The drawing under review shows one solid part. Ordinate dimensions are in mm from its lowest x, y, z. A direction names the side the tool comes from. Coordinates: 2 decimals unless noted, no trailing zeros. Write each loop counter-clockwise with the first axis right and the second up, starting at its lowest first coordinate (ties: lowest second). Pieces come first, ordered by that corner, then holes.
Q1. To check wall thickness, follow probe 1 along Y at (x, z) = (12, 112); probe 2 along Z at (x, y) = (59.3, 42). State the ranges of each line that lie inside material, in increasing order.
Q2. Add section B-B, the plane y = 42. Give the boundary of the cut face in (x, z), plus the area to 3 significant figures.
Q3. Add section A-A, the plane x = 24.5. Give the boundary of the cut face in (y, z), plus the area to 4 significant figures.
Q4. The part is to be moulded in two halves that separate along Y. For the marked faces 3, 4 and 5, say which applies: +Y half, -Y half, draft (parallel to the pull), parting line (faces both ways), or undercut.
Q5. Clearance check with flat-ended pins moving along their axes: pin 1 Ø0.9 at (x, y) = (58.5, 36) entering from -Z; pin 2 Ø2.5 at (x, y) = (28, 1.5) entering from +Z; pin 3 Ø3.5 at (x, y) = (36.5, 58.5) entering from +Z. State where each tip first meets the part, or that it passes through.
Q6. Add section D-D, the plane y = 26. Give the boundary of the cut face in (x, z).
Q7. Machinability: for the marked faces 1 and 2, which of the approach directions +Z, -Z, +X, -X, +Y, -Y give a long, thin tool a straight path to every point of the face, cutting with its end or side? Answer none if there is none.
Q8. Add section C-C, the plane z = 35. Give the boundary of the cut face in (x, y), plus the area to 3 significant figures.
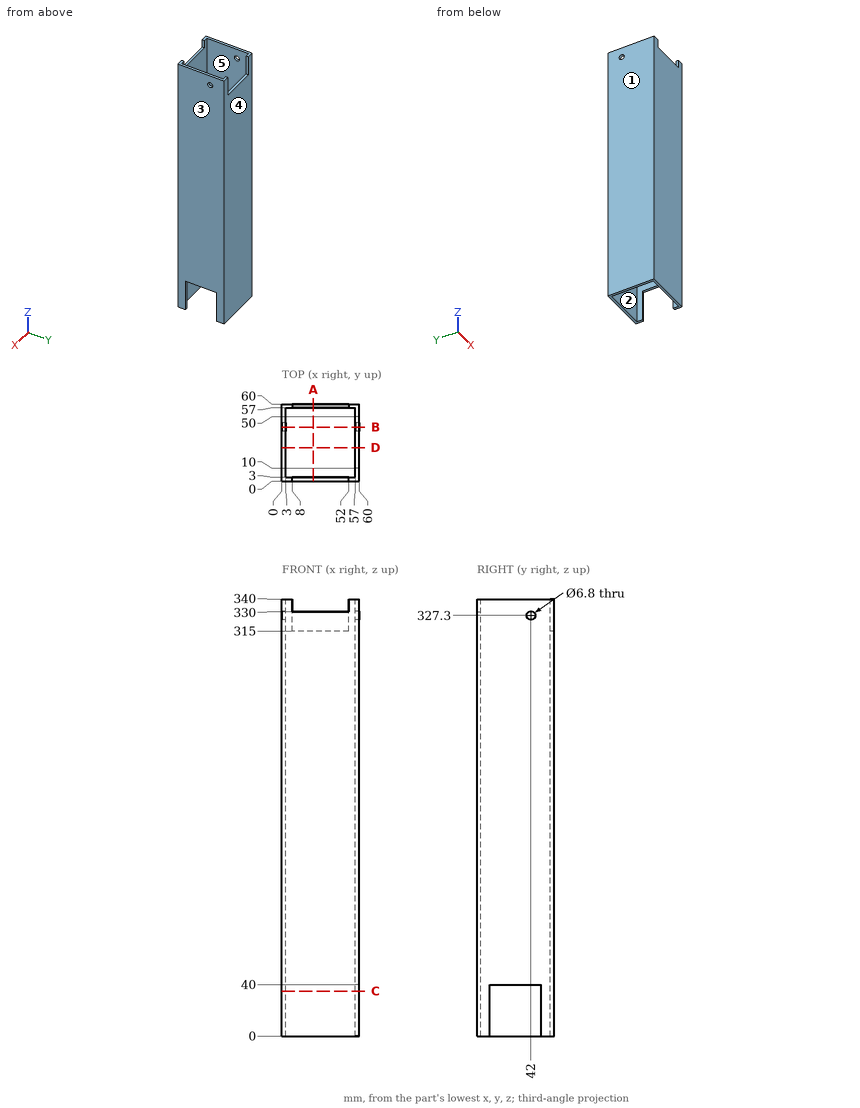
Here are the results:
1. probe 1: y = 0 to 3, 57 to 60
1. probe 2: z = 40 to 323.9, 330.7 to 340
2. outline: (0, 0) - (3, 0) - (3, 323.9) - (0, 323.9) - close; (0, 330.7) - (3, 330.7) - (3, 340) - (0, 340) - close; (57, 40) - (60, 40) - (60, 323.9) - (57, 323.9) - close; (57, 330.7) - (60, 330.7) - (60, 340) - (57, 340) - close
2. area: 1,880 mm2
3. outline: (0, 0) - (3, 0) - (3, 330) - (0, 330) - close; (57, 0) - (60, 0) - (60, 315) - (57, 315) - close
3. area: 1,935 mm2
4. face 3: draft
4. face 4: +Y half
4. face 5: undercut
5. pin 1: stops at z = 40
5. pin 2: stops at z = 330
5. pin 3: stops at z = 315
6. outline: (0, 0) - (3, 0) - (3, 340) - (0, 340) - close; (57, 40) - (60, 40) - (60, 340) - (57, 340) - close
7. face 1: +Z, -Z, -X, +Y, -Y
7. face 2: +Z, -Z
8. outline: (0, 0) - (60, 0) - (60, 10) - (57, 10) - (57, 3) - (3, 3) - (3, 57) - (57, 57) - (57, 50) - (60, 50) - (60, 60) - (0, 60) - close
8. area: 564 mm2
